from build123d import *

# Parameters (mm, degrees)
BOSS_EXTRUDE1_DEPTH = 30.7
SKETCH4_W           = 34
SKETCH4_H           = 39.4
SKETCH4_R           = 2
BOSS_EXTRUDE2_DEPTH = 2
SKETCH5_W           = 5
SKETCH5_H           = 39.4
CUT_EXTRUDE1_DEPTH  = 1
FILLET1_R           = 1
FILLET2_R           = 1
CUT_EXTRUDE2_START  = -5.95
SKETCH6_R           = 2
CUT_EXTRUDE2_DEPTH  = 5.95


with BuildPart() as part:
    # Sketch1 → Boss-Extrude1 (new, symmetric)
    with BuildSketch(Plane.XY):
        Polygon((0, 15), (0, 26), (-17, 26), (-17, 4), (-7.5, 4), (-5.5, 6), (-5.5, 9), (-7.5, 11), (-7.5, 15), align=None)
        Polygon((17, 26), (0, 26), (0, 15), (7.5, 15), (7.5, 11), (5.5, 9), (5.5, 6), (7.5, 4), (17, 4), align=None)
    extrude(amount=BOSS_EXTRUDE1_DEPTH, both=True)

    # Sketch4 → Boss-Extrude2 (add)
    with BuildSketch(Plane(origin=(0, 26, 0), x_dir=(1, 0, 0), z_dir=(0, 1, 0))):
        Rectangle(SKETCH4_W, SKETCH4_H)
        with Locations(Location((-13, 13, 0), (0, 0, 180))):
            Circle(SKETCH4_R, mode=Mode.SUBTRACT)
        with Locations((13, 13)):
            Circle(SKETCH4_R, mode=Mode.SUBTRACT)
        with Locations((-13, -13)):
            Circle(SKETCH4_R, mode=Mode.SUBTRACT)
        with Locations(Location((13, -13, 0), (0, 0, 180))):
            Circle(SKETCH4_R, mode=Mode.SUBTRACT)
    extrude(amount=BOSS_EXTRUDE2_DEPTH)

    # Sketch5 → Cut-Extrude1 (cut)
    with BuildSketch(Plane(origin=(0, 28, 0), x_dir=(1, 0, 0), z_dir=(0, 1, 0))):
        with Locations((-5.5, 0)):
            Rectangle(SKETCH5_W, SKETCH5_H)
        with Locations((5.5, 0)):
            Rectangle(SKETCH5_W, SKETCH5_H)
    extrude(amount=-CUT_EXTRUDE1_DEPTH, mode=Mode.SUBTRACT)

    # Fillet1
    fillet1_edges = [part.edges().sort_by_distance(p)[0] for p in [
        (-17, 4, 0),
        (17, 4, 0),
    ]]
    fillet(fillet1_edges, radius=FILLET1_R)

    # Fillet2
    fillet2_edges = [part.edges().sort_by_distance(p)[0] for p in [
        (-17, 15.5, -30.7),
        (17, 15.5, -30.7),
        (16.707106781, 4.292893219, -30.7),
        (-16.707106781, 4.292893219, -30.7),
        (-17, 15.5, 30.7),
        (17, 15.5, 30.7),
        (16.707106781, 4.292893219, 30.7),
        (-16.707106781, 4.292893219, 30.7),
        (-11.75, 4, -30.7),
        (0, 26, -30.7),
        (11.75, 4, -30.7),
        (11.75, 4, 30.7),
        (0, 26, 30.7),
        (-11.75, 4, 30.7),
    ]]
    fillet(fillet2_edges, radius=FILLET2_R)

    # Sketch6 → Cut-Extrude2 (cut)
    with BuildSketch(Plane(origin=(0, 28, 0), x_dir=(1, 0, 0), z_dir=(0, 1, 0)).offset(CUT_EXTRUDE2_START)):
        with Locations((-13, -13)):
            Circle(SKETCH6_R)
        with Locations(Location((13, -13, 0), (0, 0, 270))):
            Circle(SKETCH6_R)
        with Locations((13, 13)):
            Circle(SKETCH6_R)
        with Locations(Location((-13, 13, 0), (0, 0, 270))):
            Circle(SKETCH6_R)
    extrude(amount=CUT_EXTRUDE2_DEPTH, mode=Mode.SUBTRACT)


solid = part.part
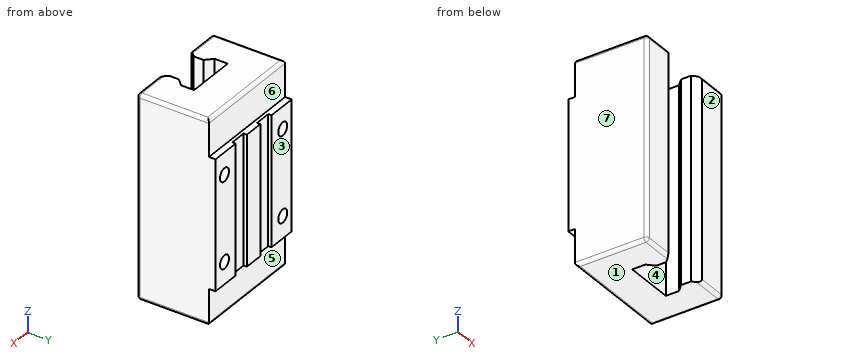
Part model, mm, in its own coordinate system. Face numbers are marked on the shaded views. A direction names the side the tool comes from. Round coordinates to 2 decimals unless told otherwise and drop trailing zeros. Write each loop counter-clockwise with the first axis right and the second up, starting at its lowest first coordinate (ties: lowest second). Pieces come first, ordered by that corner, then holes. Notation, with made-up numbers: M 78,60.25 L 112,60.25 A30 cw 112,95.25 Z; hole C 40,79 d9. An arc over 180 degrees is marked long. Return JSON: item names as keys, results as strings. Group by question number.
(1) Pin check, flat tips, straight feed: pin 1 Ø5.5 at (x, z) = (5.5, 5) entering from +Y; pin 2 Ø0.6 at (x, y) = (8.5, 27) entering from -Z; pin 3 Ø4.5 at (x, z) = (3.5, -6.5) entering from -Y; pin 4 Ø3 at (x, z) = (13, 13) entering from +Y. Stop position of each tip, or through.
(2) Drill centre lines: probe 1 along X at (y, z) = (24.25, -13); probe 2 along Z at (x, y) = (-13, 26.6); probe 3 along Z at (x, y) = (-13, 23.55). Where is each one in solid material? Low to high.
(3) Saw through at C-C on y = 12.5. Write the cut outline in (x, z).
(4) Saw through at A-A on x = -13. Write the cut outline in (y, z), then the cut area to 3 significant figures.
(5) Saw through at B-B on z = 22. Write the cut outline in (x, y).
(6) Which spindle directions (+Z, -Z, +X, -X, +Y, -Y) get a long thin tool onto all of the face, cutting with end or side? Do the marked faces 5, 6 and 7. Say none if no direction does.
(7) Two-plate mould, pull along Y, no slides. Class the marked faces 1, 2, 3 and 4: +Y half, -Y half, draft (parallel to the pull), parting line (faces both ways), or undercut.
Returned:
{
 "1": {"pin 1": "y = 28", "pin 2": "z = -19.7", "pin 3": "y = 5.75", "pin 4": "y = 22.05"},
 "2": {"probe 1": "-17 to -15, -11 to 11, 15 to 17", "probe 2": "-19.7 to -15, -11 to 11, 15 to 19.7", "probe 3": "-30.7 to -15, -11 to 11, 15 to 30.7"},
 "3": {"outline": "M -17,-29.7 A1 ccw -16,-30.7 L -7.5,-30.7 L -7.5,30.7 L -16,30.7 A1 ccw -17,29.7 Z; M 7.5,-30.7 L 16,-30.7 A1 ccw 17,-29.7 L 17,29.7 A1 ccw 16,30.7 L 7.5,30.7 Z"},
 "4": {"outline": "M 4,-29.7 A1 ccw 5,-30.7 L 25,-30.7 A1 ccw 26,-29.7 L 26,-19.7 L 28,-19.7 L 28,-15 L 22.05,-15 L 22.05,-11 L 28,-11 L 28,11 L 22.05,11 L 22.05,15 L 28,15 L 28,19.7 L 26,19.7 L 26,29.7 A1 ccw 25,30.7 L 5,30.7 A1 ccw 4,29.7 Z", "area": "1,380 mm²"},
 "5": {"outline": "M -17,5 A1 ccw -16,4 L -7.5,4 L -5.5,6 L -5.5,9 L -7.5,11 L -7.5,15 L 7.5,15 L 7.5,11 L 5.5,9 L 5.5,6 L 7.5,4 L 16,4 A1 ccw 17,5 L 17,26 L -17,26 Z"},
 "6": {"face 5": "-Z, +X, -X, +Y", "face 6": "+Z, +X, -X, +Y", "face 7": "+Z, -Z, -X, +Y, -Y"},
 "7": {"face 1": "draft", "face 2": "-Y half", "face 3": "+Y half", "face 4": "undercut"}
}
